Work out the finished part from the listing and answer in its coordinate system (mm). Face numbers are marked on the shaded views. Coordinates: 2 decimals unless noted, no trailing zeros. Write each loop counter-clockwise with the first axis right and the second up, starting at its lowest first coordinate (ties: lowest second). Pieces come first, ordered by that corner, then holes. Notation, with made-up numbers: (69.5, 5.25) - (103.5, 5.25) arc R26 ccw to (103.5, 29.25) - close; hole circle Ø4 at (77.25, 37.25). An arc over 180 degrees is marked (long way). Use a Markdown table: item, result. Add a question column.
(1) The part is cut by section C-C, the plane z = 1. Give the vertices of the cut face in (x, y), then the cut area to 3 significant figures.
(2) The part is cut by section D-D, the plane y = 0. State how many separate pieces and enclosed holes the cut face has, then the cut area to 3 significant figures.
(3) For a pull along X with two mould halves and no side action, classify the marked faces 1 and 2 as released by +X, released by -X, zero draft, split by the parting line, or undercut.
(4) Find the intervals of material crossed by line 1 (Y direction, x = -17, z = 1.15); line 2 (X direction, y = 0, z = 2.6); line 3 (Y direction, x = -16, z = 13.5), in increasing order. Write a range as from..to.
(5) The part is cut by section A-A, the plane z = 8.5. Give the vertices of the cut face in (x, y).
(6) Given pin 1 Ø10 at (x, y) = (22, 10) entering from -Z; pin 2 Ø9 at (y, z) = (7.5, 8) entering from -X; pin 3 Ø13.5 at (x, y) = (0, 0) entering from -Z; pin 4 Ø4 at (x, z) = (21.5, 7.5) entering from -Y, each flat-ended and moving along its own axis, determine where each tip first touches the part or whether it passes through.
(7) The part is cut by section B-B, the plane x = 0. Give the vertices of the cut face in (y, z), then the cut area to 3 significant figures.
from build123d import *

# Parameters (mm, degrees)
EXTRUDE_1_DEPTH     = 3
SKETCH_2_R          = 1.6
SKETCH_2_R_2        = 2.55
CUT_EXTRUDE_1_DEPTH = 5
EXTRUDE_START       = 8
SKETCH_3_R          = 4
SKETCH_3_R_2        = 2.55
EXTRUDE_2_DEPTH     = 8
EXTRUDE_4_DEPTH     = 3
EXTRUDE_5_REACH     = 41
SKETCH_6_W          = 20
SKETCH_6_H          = 44.72135955
SKETCH_8_R          = 1.6
CUT_EXTRUDE_6_DEPTH = 10
SKETCH_9_R          = 3
CUT_EXTRUDE_7_DEPTH = 20
SKETCH_10_R         = 11.1
CUT_EXTRUDE_8_DEPTH = 2.1
SKETCH_11_R         = 5
SKETCH_11_R_2       = 3
EXTRUDE_6_DEPTH     = 2.4
FILLET_1_R          = 0.5
SKETCH_12_R         = 2.55
EXTRUDE_7_DEPTH     = 5


with BuildPart() as part:
    # 草图1 → 凸台-拉伸1 (new body)
    with BuildSketch(Plane.XY):
        with BuildLine():
            Line((-20, 22.360679775), (20, 22.360679775))
            ThreePointArc((20, 22.360679775), (30, 0), (20, -22.360679775))
            Line((20, -22.360679775), (-20, -22.360679775))
            ThreePointArc((-20, -22.360679775), (-30, 0), (-20, 22.360679775))
        make_face()
    extrude(amount=EXTRUDE_1_DEPTH)

    # 草图2 → 切除-拉伸1 (cut)
    with BuildSketch(Plane.XY.offset(3)):
        with Locations((17, 8)):
            Circle(SKETCH_2_R)
        with Locations((-17, 0)):
            Circle(SKETCH_2_R_2)
        with Locations((17, 0)):
            Circle(SKETCH_2_R_2)
        with Locations((17, -8)):
            Circle(SKETCH_2_R)
        with Locations((-17, -8)):
            Circle(SKETCH_2_R)
        with Locations((-17, 8)):
            Circle(SKETCH_2_R)
    extrude(amount=-CUT_EXTRUDE_1_DEPTH, mode=Mode.SUBTRACT)

    # 草图3 → 凸台-拉伸2 (add)
    # profile 1 of 2: a face of its own
    with BuildSketch(Plane.XY.offset(3).offset(EXTRUDE_START)):
        with Locations((17, 0)):
            Circle(SKETCH_3_R)
        with Locations((17, 0)):
            Circle(SKETCH_3_R_2, mode=Mode.SUBTRACT)
    # profile 2 of 2: a face of its own
    with BuildSketch(Plane.XY.offset(3).offset(EXTRUDE_START)):
        with Locations((-17, 0)):
            Circle(SKETCH_3_R)
        with Locations((-17, 0)):
            Circle(SKETCH_3_R_2, mode=Mode.SUBTRACT)
    extrude(amount=-EXTRUDE_2_DEPTH)

    # 草图5 → 凸台-拉伸4 (add)
    with BuildSketch(Plane.XY.offset(11)):
        with BuildLine():
            Line((-20, -22.360679775), (20, -22.360679775))
            ThreePointArc((20, -22.360679775), (30, 0), (20, 22.360679775))
            Line((20, 22.360679775), (-20, 22.360679775))
            ThreePointArc((-20, 22.360679775), (-30, 0), (-20, -22.360679775))
        make_face()
    extrude(amount=EXTRUDE_4_DEPTH)

    # 草图6 → 凸台-拉伸5 (add, up to next)
    with BuildSketch(Plane.XY.offset(3), mode=Mode.PRIVATE) as extrude_5_sk1:
        Rectangle(SKETCH_6_W, SKETCH_6_H)
    extrude_5_tool1 = extrude(extrude_5_sk1.sketch, amount=EXTRUDE_5_REACH, mode=Mode.PRIVATE) - part.part
    add(extrude_5_tool1.solids().sort_by_distance((0, 0, 3))[0])

    # 草图8 → 切除-拉伸6 (cut)
    with BuildSketch(Plane.XY.offset(14)):
        with Locations((15.5, 15.5)):
            Circle(SKETCH_8_R)
        with Locations((15.5, -15.5)):
            Circle(SKETCH_8_R)
        with Locations((-15.5, -15.5)):
            Circle(SKETCH_8_R)
        with Locations((-15.5, 15.5)):
            Circle(SKETCH_8_R)
    extrude(amount=-CUT_EXTRUDE_6_DEPTH, mode=Mode.SUBTRACT)

    # 草图9 → 切除-拉伸7 (cut)
    with BuildSketch(Plane.XY.offset(14)):
        Circle(SKETCH_9_R)
    extrude(amount=-CUT_EXTRUDE_7_DEPTH, mode=Mode.SUBTRACT)

    # 草图10 → 切除-拉伸8 (cut)
    with BuildSketch(Plane.XY.offset(14)):
        Circle(SKETCH_10_R)
    extrude(amount=-CUT_EXTRUDE_8_DEPTH, mode=Mode.SUBTRACT)

    # 草图11 → 凸台-拉伸6 (add)
    with BuildSketch(Plane(origin=(0, 0, 0), x_dir=(-1, 0, 0), z_dir=(0, 0, -1))):
        with Locations(Location((0, 0, 0), (0, 0, 180))):
            Circle(SKETCH_11_R)
        with Locations(Location((0, 0, 0), (0, 0, 180))):
            Circle(SKETCH_11_R_2, mode=Mode.SUBTRACT)
    extrude(amount=EXTRUDE_6_DEPTH)

    # 圆角1
    fillet_1_edges = [part.edges().sort_by_distance(p)[0] for p in [
        (-5, 0, 0),
        (-3, 0, -2.4),
        (-5, 0, -2.4),
    ]]
    fillet(fillet_1_edges, radius=FILLET_1_R)

    # 草图12 → 凸台-拉伸7 (add)
    with BuildSketch(Plane(origin=(0, 0, 11), x_dir=(-1, 0, 0), z_dir=(0, 0, -1))):
        with Locations(Location((-17, 0, 0), (0, 0, 180))):
            Circle(SKETCH_12_R)
        with Locations(Location((17, 0, 0), (0, 0, 180))):
            Circle(SKETCH_12_R)
    extrude(amount=EXTRUDE_7_DEPTH)


solid = part.part
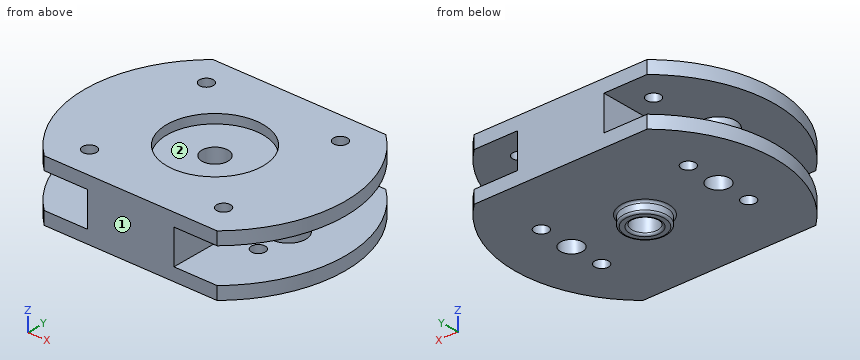
Model answer:
| question | item | result |
|---|---|---|
| 1 | outline | (-20, -22.36) - (20, -22.36) arc R30 ccw to (20, 22.36) - (-20, 22.36) arc R30 ccw to start; hole circle Ø5.1 at (-17, 0); hole circle Ø3.2 at (-17, -8); hole circle Ø3.2 at (-17, 8); hole circle Ø6 at (0, 0); hole circle Ø5.1 at (17, 0); hole circle Ø3.2 at (17, -8); hole circle Ø3.2 at (17, 8) |
| 1 | area | 2,310 mm^2 |
| 2 | separate pieces | 2 |
| 2 | enclosed holes | 2 |
| 2 | area | 478 mm^2 |
| 3 | face 1 | zero draft |
| 3 | face 2 | undercut |
| 4 | line 1 | -22.36..-9.6, -6.4..-2.55, 2.55..6.4, 9.6..22.36 |
| 4 | line 2 | -30..-19.55, -14.45..-3, 3..14.45, 19.55..30 |
| 4 | line 3 | -22.36..-17.02, -13.98..13.98, 17.02..22.36 |
| 5 | outline | circle Ø8 at (-17, 0); (-10, -22.36) - (10, -22.36) - (10, 22.36) - (-10, 22.36) - close; circle Ø8 at (17, 0); hole circle Ø6 at (0, 0) |
| 6 | pin 1 | z = 0 |
| 6 | pin 2 | x = -29.71 |
| 6 | pin 3 | z = -2.4 |
| 6 | pin 4 | y = -3.12 |
| 7 | outline | (-22.36, 0) - (-5.5, 0) arc R0.5 cw to (-5, -0.5) - (-5, -1.9) arc R0.5 ccw to (-4.5, -2.4) - (-3.5, -2.4) arc R0.5 ccw to (-3, -1.9) - (-3, 11.9) - (-11.1, 11.9) - (-11.1, 14) - (-22.36, 14) - close; (3, -1.9) arc R0.5 ccw to (3.5, -2.4) - (4.5, -2.4) arc R0.5 ccw to (5, -1.9) - (5, -0.5) arc R0.5 cw to (5.5, 0) - (22.36, 0) - (22.36, 14) - (11.1, 14) - (11.1, 11.9) - (3, 11.9) - close |
| 7 | area | 518 mm^2 |
